The model under review builds one solid part; all positions refer to its coordinate system, in mm. A direction names the side the tool comes from. Round coordinates to 2 decimals unless told otherwise and drop trailing zeros. Loops run counter-clockwise (first coordinate to the right, second up) from the corner with the lowest first, then second, coordinate; pieces in that order, holes last. Notation, with made-up numbers: M -25.5,60.25 L 18.5,60.25 A15 ccw 18.5,82.25 Z; hole C -37,-23 d2. An arc over 180 degrees is marked long. Answer as a JSON object with one key per item and string values. Group by question number.
Item 1: Consider section A-A (x = -6). Give the boundary of the cut face in (y, z), and give its area (3 significant figures).
Item 2: Tool access review of faces 4 (the face through (16.897, 113, 20)), 5 (the face through (-1.369, 217.394, 37.972)), 6 (the face through (-19.103, 111, 20)): name each direction out of +Z, -Z, +X, -X, +Y, -Y from which nothing blocks a thin tool from reaching the whole face with its end or side.
Item 3: The part is to be moulded in two halves that separate along X. For faces 1 (the face through (-1.69, 231.55, 2.03)), 2 (the face through (-3, 117, 40)), 3 (the face through (-23.103, 113, 20)), say which applies: +X half, -X half, draft (parallel to the pull), parting line (faces both ways), or undercut.
Item 4: Insertion check: P1, Ø14.5, axis at x = -3.1, y = 225.2, coming from the +Z side; P2, Ø1, axis at x = -1, y = 20.5, coming from the -Z side. Each pin has a flat end and moves straight along its axis. Give the tip position at first contact, or say it passes through.
Item 5: Consider section B-B (z = 10). Give the boundary of the cut face in (x, y).
Item 6: To check wall thickness, follow line 1 (Z direction, x = -13.5, y = -21.5); line 2 (X direction, y = 186, z = 18); line 3 (Y direction, x = 6, z = 26.5). State the ranges of each line that lie inside material, in increasing order.
Item 7: Consider section C-C (y = 157). Give the boundary of the cut face in (x, z), and give its area (3 significant figures).
```python
from build123d import *

# Parameters (mm, degrees)
F0_W     = 40
F0_H     = 300
F1_DEPTH = 40
F2_T     = -4
F4_D     = 16
F4_DEPTH = 4
F6_D     = 13
F6_DEPTH = 4


with BuildPart() as f1:
    # F0 (on Top) → F1 (new body)
    with BuildSketch(Plane.XY):
        with Locations((-3.103449, 115.204206)):
            Rectangle(F0_W, F0_H)
    extrude(amount=F1_DEPTH)

    # F2
    f2_openings = [f1.faces().sort_by_distance(p)[0] for p in [
        (-3.103449, -34.795794, 20),
    ]]
    offset(amount=F2_T, openings=f2_openings)

    # F4
    with Locations(Plane.XY.offset(40)):
        with Locations((-3.103449, 225.204206)):
            Hole(F4_D / 2, depth=F4_DEPTH)

    # F6
    with Locations(Plane(origin=(0, 0, 0), x_dir=(1, 0, 0), z_dir=(0, 0, -1))):
        with Locations((-3.103449, -225.204206)):
            Hole(F6_D / 2, depth=F6_DEPTH)


solid = f1.part
```
Geometry results:
{
 "1": {"outline": "M -34.8,0 L 219.39,0 L 219.39,4 L -34.8,4 Z; M -34.8,36 L 217.75,36 L 217.75,40 L -34.8,40 Z; M 231.02,0 L 265.2,0 L 265.2,40 L 232.66,40 L 232.66,36 L 261.2,36 L 261.2,4 L 231.02,4 Z", "area": "2,420 mm^2"},
 "2": {"face 4": "+Z, -Z, +X, +Y, -Y", "face 5": "+Z", "face 6": "-Y"},
 "3": {"face 1": "undercut", "face 2": "draft", "face 3": "-X half"},
 "4": {"P1": "stops at z = 4", "P2": "stops at z = 0"},
 "5": {"outline": "M -23.1,-34.8 L -19.1,-34.8 L -19.1,261.2 L 12.9,261.2 L 12.9,-34.8 L 16.9,-34.8 L 16.9,265.2 L -23.1,265.2 Z"},
 "6": {"line 1": "z = 0 to 4, 36 to 40", "line 2": "x = -23.1 to -19.1, 12.9 to 16.9", "line 3": "y = 261.2 to 265.2"},
 "7": {"outline": "M -23.1,0 L 16.9,0 L 16.9,40 L -23.1,40 Z; hole M -19.1,4 L 12.9,4 L 12.9,36 L -19.1,36 Z", "area": "576 mm^2"}
}
